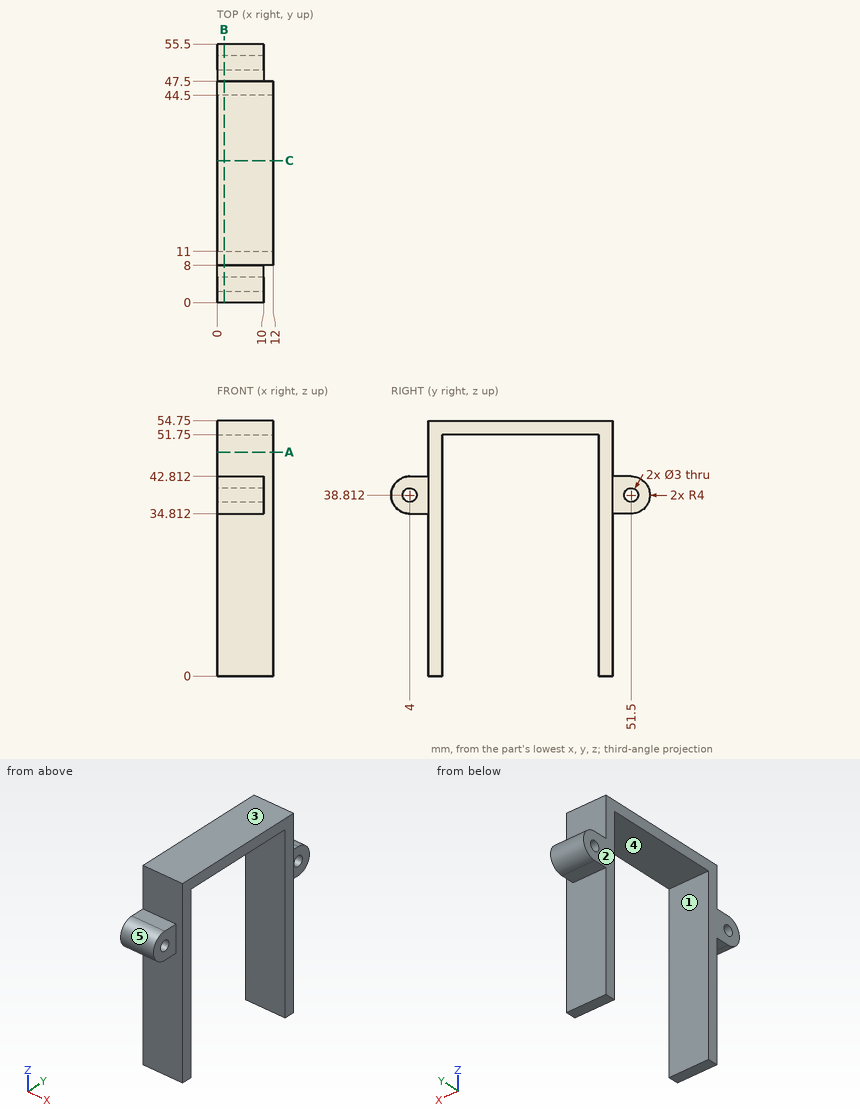
Drawing for the job (mm, zero at the part's lowest x, y, z). A direction names the side the tool comes from. Round coordinates to 2 decimals unless told otherwise and drop trailing zeros. Write each loop counter-clockwise with the first axis right and the second up, starting at its lowest first coordinate (ties: lowest second). Pieces come first, ordered by that corner, then holes. Notation, with made-up numbers: M 67,80.25 L 120,80.25 A18 cw 120,94.25 Z; hole C 67,86.5 d2. An arc over 180 degrees is marked long. Answer as a JSON object with one key per item and string values. Group by question number.
(1) Cut at B-B (x = 1.5). Give the cut face in (y, z).
(2) Cut at A-A (z = 48). Give the cut face in (x, y).
(3) Which spindle directions (+Z, -Z, +X, -X, +Y, -Y) get a long thin tool onto all of the face, cutting with end or side? Do the marked faces 1 and 2. Say none if no direction does.
(4) Cut at C-C (y = 30.5). Give the cut face in (x, z), and give its area (3 significant figures).
(5) Drill centre lines: L1, parallel to Y at x = 4.5, z = 49; L2, parallel to Z at x = 2.5, y = 51.5; L3, parallel to Z at x = 4, y = 36.5. Where is each one in solid material? Low to high.
(6) Mould opens along Y. For the marked faces 3, 4 and 5 say: pulls with the +Y half, pulls with the -Y half, needs draft (parallel to the pull), parting line crosses it, or undercut.
(7) Flat gauge pins, fed straight in: pin 1 (1.5 mm diameter, centred on x = 4, z = 10, fed in from +Y); pin 2 (12 mm diameter, centred on y = 34, z = 36, fed in from +X); pin 3 (6.5 mm diameter, centred on y = 50.5, z = 40.5, fed in from +X); pin 4 (1.2 mm diameter, centred on x = 6, y = 6.5, fed in from +Z). Where does each tip first touch, or does it go through?
Responses:
{
 "1": {"outline": "M 4,34.81 L 8,34.81 L 8,0 L 11,0 L 11,51.75 L 44.5,51.75 L 44.5,0 L 47.5,0 L 47.5,34.81 L 51.5,34.81 A4 ccw 51.5,42.81 L 47.5,42.81 L 47.5,54.75 L 8,54.75 L 8,42.81 L 4,42.81 A4 ccw Z; hole C 4,38.81 d3; hole C 51.5,38.81 d3"},
 "2": {"outline": "M 0,8 L 12,8 L 12,11 L 0,11 Z; M 0,44.5 L 12,44.5 L 12,47.5 L 0,47.5 Z"},
 "3": {"face 1": "-Z, +X, -X", "face 2": "+Z, -Z, -X, +Y, -Y"},
 "4": {"outline": "M 0,51.75 L 12,51.75 L 12,54.75 L 0,54.75 Z", "area": "36.0 mm2"},
 "5": {"L1": "y = 8 to 11, 44.5 to 47.5", "L2": "z = 34.81 to 37.31, 40.31 to 42.81", "L3": "z = 51.75 to 54.75"},
 "6": {"face 3": "needs draft", "face 4": "undercut", "face 5": "pulls with the -Y half"},
 "7": {"pin 1": "stops at y = 47.5", "pin 2": "passes through", "pin 3": "stops at x = 12", "pin 4": "stops at z = 42.81"}
}
